CAD build for the part. Positions are in the model's coordinates, mm. Face numbers are marked on the shaded views. A direction names the side the tool comes from. Round coordinates to 2 decimals unless told otherwise and drop trailing zeros. Order: outer loops, then holes, each group sorted by start corner. A loop starts at its lowest first (then second) coordinate and runs counter-clockwise, first axis right, second up. Notation, with made-up numbers: (-21.5, 56) - (28.5, 56) arc R32 ccw to (28.5, 89) - close; hole circle Ø1 at (-23.5, -2). An arc over 180 degrees is marked (long way). Write item = value, one per line.
from build123d import *

# Parameters (mm, degrees)
BOSS_EXTRUDE1_DEPTH = 12.5
FILLET1_R           = 3
SKETCH2_R           = 1.75
CUT_EXTRUDE1_DEPTH  = 15.361406616
SKETCH3_R           = 1.75
CUT_EXTRUDE2_DEPTH  = 17.007810594


with BuildPart() as part:
    # Sketch1 → Boss-Extrude1 (new, symmetric)
    with BuildSketch(Plane.XY):
        Polygon((-3, 1), (5, 1), (5, -1), (-5, -1), (-5, 1), (-5, 6), (-3, 6), align=None)
    extrude(amount=BOSS_EXTRUDE1_DEPTH, both=True)

    # Fillet1
    fillet1_edges = [part.edges().sort_by_distance(p)[0] for p in [
        (5, 0, -12.5),
        (-4, 6, 12.5),
        (5, 0, 12.5),
        (-4, 6, -12.5),
    ]]
    fillet(fillet1_edges, radius=FILLET1_R)

    # Sketch2 → Cut-Extrude1 (cut, through all)
    with BuildSketch(Plane(origin=(0, 1, 0), x_dir=(1, 0, 0), z_dir=(0, 1, 0))):
        with Locations(Location((2, -9.5, 0), (0, 0, 270))):
            Circle(SKETCH2_R)
        with Locations(Location((2, 9.5, 0), (0, 0, 90))):
            Circle(SKETCH2_R)
    extrude(amount=-CUT_EXTRUDE1_DEPTH, mode=Mode.SUBTRACT)

    # Sketch3 → Cut-Extrude2 (cut, through all)
    with BuildSketch(Plane(origin=(-3, 0, 0), x_dir=(0, 0, -1), z_dir=(1, 0, 0))):
        with Locations((0, 3.5)):
            Circle(SKETCH3_R)
    extrude(amount=-CUT_EXTRUDE2_DEPTH, mode=Mode.SUBTRACT)


solid = part.part
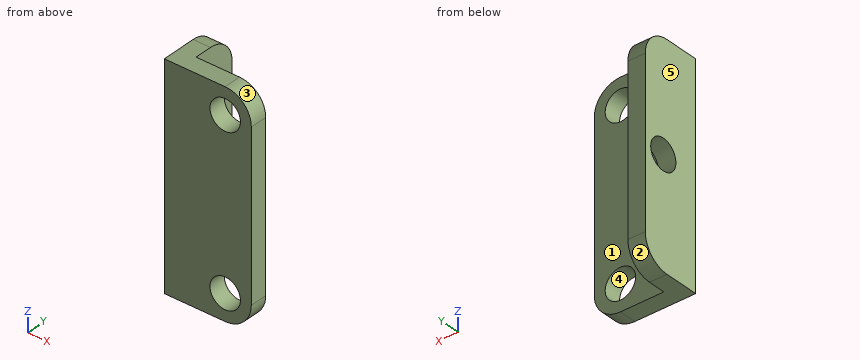
(1) Band-saw the part on C-C on y = 4.5. List the corners of the cut face in (x, z).
Solved:
outline = (-5, -12.1) - (-3, -12.1) - (-3, -1.44) - (-5, -1.44) - close; (-5, 1.44) - (-3, 1.44) - (-3, 12.1) - (-5, 12.1) - close
(2) Band-saw the part on D-D on x = 3. List the corners of the cut face in (y, z).
Solved:
outline = (-1, -12.33) - (1, -12.33) - (1, -10.94) - (-1, -10.94) - close; (-1, -8.06) - (1, -8.06) - (1, 8.06) - (-1, 8.06) - close; (-1, 10.94) - (1, 10.94) - (1, 12.33) - (-1, 12.33) - close
(3) Band-saw the part on A-A on z = 0. List the corners of the cut face in (x, y), plus the area to 3 significant figures.
Solved:
outline = (-5, -1) - (5, -1) - (5, 1) - (-3, 1) - (-3, 1.75) - (-5, 1.75) - close; (-5, 5.25) - (-3, 5.25) - (-3, 6) - (-5, 6) - close
area = 23.0 mm²
(4) Band-saw the part on B-B on x = -3.25. List the corners of the cut face in (y, z), plus the area to 3 significant figures.
Solved:
outline = (-1, -12.5) - (3, -12.5) arc R3 ccw to (6, -9.5) - (6, 9.5) arc R3 ccw to (3, 12.5) - (-1, 12.5) - close; hole circle Ø3.5 at (3.5, 0)
area = 162 mm²
(5) Drop flat-ended pins along their axis: pin 1 (4 mm diameter, centred on x = 2, z = 9.5, fed in from +Y); pin 2 (4 mm diameter, centred on x = 2.5, y = 0, fed in from -Z); pin 3 (1.5 mm diameter, centred on y = 2.5, z = 1, fed in from +X). Give the stop position or say it passes through.
Solved:
pin_1 = 1
pin_2 = -12.5
pin_3 = -3
(6) Probe line 1 along X through (y, z) = (-0.25, -9.5); line 2 along Y through (x, z) = (-4.2, 0); line 3 along X through (y, z) = (1.25, -8.5). List the from-to ranges inside material, lowest first.
Solved:
line_1 = -5 to 0.25, 3.75 to 5
line_2 = -1 to 1.75, 5.25 to 6
line_3 = -5 to -3
(7) Tool access for the marked faces 1 and 2: list every direction of +Z, -Z, +X, -X, +Y, -Y with a clear straight run to the whole face (end or side of a thin tool).
Solved:
face_1 = +Z, -Z, +X, +Y
face_2 = -Z, +X, -X, +Y
(8) Pull direction X, two halves, no side cores. Call the marked faces 3, 4 and 5: released by +X, released by -X, zero draft, split by the parting line, or undercut.
Solved:
face_3 = released by +X
face_4 = undercut
face_5 = released by -X
